from build123d import *

# Parameters (mm, degrees)
F1_DEPTH = 50


with BuildPart() as f1:
    # F0 (on Front) → F1 (new body, symmetric)
    with BuildSketch(Plane.XZ):
        Polygon((19.9459, -8), (19.9459, 10), (17.6872, 10), (17.6872, -8), (13.6872, -8), (13.6872, 10), (11.4285, 10), (11.4285, -8), (7.4285, -8), (7.4285, 10), (5.1428, 10), (5.1428, -8), (1.1428, -8), (1.1428, 10), (-1.1429, 10), (-1.1429, -8), (-5.1429, -8), (-5.1429, 10), (-7.4286, 10), (-7.4286, -8), (-11.4286, -8), (-11.4286, 10), (-13.7143, 10), (-13.7143, -8), (-17.7143, -8), (-17.7143, 10), (-20, 10), (-20, -10), (19.9459, -10), align=None)
    extrude(amount=F1_DEPTH, both=True)


solid = f1.part
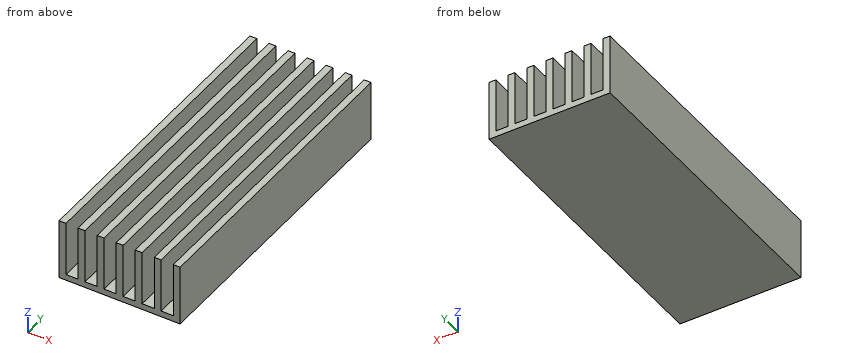
Input: part model. Units: mm. Frame: model coordinates. Coordinates: 2 decimals unless noted, no trailing zeros. Loops run counter-clockwise (first coordinate to the right, second up) from the corner with the lowest first, then second, coordinate; pieces in that order, holes last.
(1) Section C-C on x = -16. Return the cut outline in (y, z).
(2) Section A-A on z = -3.25. Return the cut outline in (x, y).
(3) Material intervals for probe 1 along Z at (x, y) = (10, -16), sorted ascending.
(4) Section B-B on y = -12.5. Return the cut outline in (x, z), then the cut area to 3 significant figures.
(5) First-contact query: pin 1 Ø2 at (x, y) = (15, 22) entering from +Z. Flat tip, straight axial feed; report the tip coordinate or a pass-through.
Data:
1. outline: (-50, -10) - (50, -10) - (50, -8) - (-50, -8) - close
2. outline: (-20, -50) - (-17.71, -50) - (-17.71, 50) - (-20, 50) - close; (-13.71, -50) - (-11.43, -50) - (-11.43, 50) - (-13.71, 50) - close; (-7.43, -50) - (-5.14, -50) - (-5.14, 50) - (-7.43, 50) - close; (-1.14, -50) - (1.14, -50) - (1.14, 50) - (-1.14, 50) - close; (5.14, -50) - (7.43, -50) - (7.43, 50) - (5.14, 50) - close; (11.43, -50) - (13.69, -50) - (13.69, 50) - (11.43, 50) - close; (17.69, -50) - (19.95, -50) - (19.95, 50) - (17.69, 50) - close
3. probe 1: z = -10 to -8
4. outline: (-20, -10) - (19.95, -10) - (19.95, 10) - (17.69, 10) - (17.69, -8) - (13.69, -8) - (13.69, 10) - (11.43, 10) - (11.43, -8) - (7.43, -8) - (7.43, 10) - (5.14, 10) - (5.14, -8) - (1.14, -8) - (1.14, 10) - (-1.14, 10) - (-1.14, -8) - (-5.14, -8) - (-5.14, 10) - (-7.43, 10) - (-7.43, -8) - (-11.43, -8) - (-11.43, 10) - (-13.71, 10) - (-13.71, -8) - (-17.71, -8) - (-17.71, 10) - (-20, 10) - close
4. area: 367 mm2
5. pin 1: stops at z = -8
